from build123d import *

# Parameters (mm, degrees)
SKICA1_W                 = 36
SKICA1_H                 = 21
P_IDAT_VYSUNUT_M1_DEPTH  = 15
SKICA2_W                 = 40.125032636
SKICA2_H                 = 25.475200522
SKICA2_W_2               = 26
SKICA2_H_2               = 18
ODEBRAT_VYSUNUT_M1_DEPTH = 3
SKICA3_R                 = 4
P_IDAT_VYSUNUT_M2_DEPTH  = 14
SKICA4_W                 = 4.119571066
SKICA4_H                 = 0.8
P_IDAT_VYSUNUT_M3_DEPTH  = 1
ZAOBLIT3_R               = 0.3


with BuildPart() as part:
    # Skica1 → Přidat vysunutím1 (new body)
    with BuildSketch(Plane.XY):
        Rectangle(SKICA1_W, SKICA1_H)
    extrude(amount=P_IDAT_VYSUNUT_M1_DEPTH)

    # Skica2 → Odebrat vysunutím1 (cut)
    with BuildSketch(Plane.XY.offset(15)):
        Rectangle(SKICA2_W, SKICA2_H)
        Rectangle(SKICA2_W_2, SKICA2_H_2, mode=Mode.SUBTRACT)
    extrude(amount=-ODEBRAT_VYSUNUT_M1_DEPTH, mode=Mode.SUBTRACT)

    # Skica3 → Přidat vysunutím2 (add)
    with BuildSketch(Plane.ZY.offset(18)):
        with Locations((13.3, 4.3)):
            Circle(SKICA3_R)
    extrude(amount=P_IDAT_VYSUNUT_M2_DEPTH)

    # Skica4 → Přidat vysunutím3 (add)
    with BuildSketch(Plane.XY.offset(12)):
        with Locations((-15.940214467, 6.8)):
            Rectangle(SKICA4_W, SKICA4_H)
        with Locations((-15.940214467, 4.3)):
            Rectangle(SKICA4_W, SKICA4_H)
        with Locations((-15.940214467, 1.8)):
            Rectangle(SKICA4_W, SKICA4_H)
    extrude(amount=P_IDAT_VYSUNUT_M3_DEPTH)

    # Zaoblit3
    zaoblit3_edges = [part.edges().sort_by_distance(p)[0] for p in [
        (13, 0, 15),
        (13, -9, 13.5),
        (0, -9, 15),
        (-13, -9, 13.5),
        (-13, 0, 15),
        (-13, 9, 13.5),
        (0, 9, 15),
        (13, 9, 13.5),
        (-13.880428934, 6.4, 12.5),
        (-13.880428934, 7.2, 12.5),
        (-15.940214467, 6.4, 13),
        (-13.880428934, 6.8, 13),
        (-15.940214467, 7.2, 13),
        (-13.880428934, 4.7, 12.5),
        (-13.880428934, 3.9, 12.5),
        (-15.940214467, 4.7, 13),
        (-15.940214467, 3.9, 13),
        (-13.880428934, 4.3, 13),
    ]]
    fillet(zaoblit3_edges, radius=ZAOBLIT3_R)


solid = part.part
Source: CAD feature listing. Evaluate the final solid. Frame: model axes, mm. A direction names the side the tool comes from. Give positions to 0.01 mm unless a question says otherwise; leave off trailing zeros. Write each loop counter-clockwise with the first axis right and the second up, starting at its lowest first coordinate (ties: lowest second). Pieces come first, ordered by that corner, then holes. Notation, with made-up numbers: M -15,70 L 44,70 A21 cw 44,107 Z; hole C -7.5,76.5 d7. An arc over 180 degrees is marked long. Return JSON: item names as keys, results as strings. Group by question number.
1) Cut plane D-D, the plane y = 2.75. Output: boundary loops of the cut face in (x, z).
2) Material intervals for line 1 along X through (y, z) = (9.5, 9.25); line 2 along Z through (x, y) = (-11.5, 7.5); line 3 along Z through (x, y) = (-20, 4.25), sorted ascending. Write a range as [from, to].
3) Pin query (flat end, axial travel): P1, Ø1.1, axis at x = -17, z = 12.5, coming from the +Y side; P2, Ø5, axis at x = -21.5, z = 8, coming from the +Y side; P3, Ø3.5, axis at y = 3, z = 5.5, coming from the -X side; P4, Ø8.5, axis at x = -3.5, y = -0.5, coming from the +Z side. Return the tip coordinate at first contact, or that it passes through.
4) Cut plane A-A, the plane y = -1.75. Output: boundary loops of the cut face in (x, z).
5) Pull-direction query (X, two-part tool) for faces 1 (the face through (-18, 4, 15)), 2 (the face through (-18, 0, 6)), 3 (the face through (0, 9, 13)); classes: pulls with the +X half, pulls with the -X half, needs draft (parallel to the pull), parting line crosses it, or undercut.
6) Cut plane C-C, the plane z = 2. Output: boundary loops of the cut face in (x, y), plus the area to 3 significant figures.
7) Set-up query: faces 4 (the face through (-0.3, -9.2, 12)), 5 (the face through (-16, 1.4, 12.5)), 6 (the face through (-24.9, 1.9, 10.1)), 7 (the face through (13, 0, 13)), 8 (the face through (-13, 0, 13)). Return all of +Z, -Z, +X, -X, +Y, -Y with unobstructed straight access to the full face (end or side cutting, diameter ignored); none if empty.
8) Cut plane B-B, the plane x = -12. Output: boundary loops of the cut face in (y, z).
Recorded:
{
 "1": {"outline": "M -32,9.61 L -18,9.61 L -18,0 L 18,0 L 18,12 L 13,12 L 13,14.7 A0.3 ccw 12.7,15 L -12.7,15 A0.3 ccw -13,14.7 L -13,12 L -18,12 L -18,16.99 L -32,16.99 Z"},
 "2": {"line 1": "x = [-18, 18]", "line 2": "z = [0, 15]", "line 3": "z = [9.3, 17.3]"},
 "3": {"P1": "stops at y = 10.5", "P2": "stops at y = 7.16", "P3": "stops at x = -18", "P4": "stops at z = 15"},
 "4": {"outline": "M -18,0 L 18,0 L 18,12 L 13,12 L 13,14.7 A0.3 ccw 12.7,15 L -12.7,15 A0.3 ccw -13,14.7 L -13,12 L -18,12 Z"},
 "5": {"face 1": "undercut", "face 2": "pulls with the -X half", "face 3": "needs draft"},
 "6": {"outline": "M -18,-10.5 L 18,-10.5 L 18,10.5 L -18,10.5 Z", "area": "756 mm²"},
 "7": {"face 4": "+Z", "face 5": "+Z, -Y", "face 6": "-X", "face 7": "+Z, +X, +Y, -Y", "face 8": "+Z, +Y, -Y"},
 "8": {"outline": "M -10.5,0 L 10.5,0 L 10.5,12 L 9,12 L 9,14.7 A0.3 ccw 8.7,15 L -8.7,15 A0.3 ccw -9,14.7 L -9,12 L -10.5,12 Z"}
}
